The listing builds one solid part. Answer for the finished solid, in the listing's coordinates (mm). Coordinates: 2 decimals unless noted, no trailing zeros. Order: outer loops, then holes, each group sorted by start corner. A loop starts at its lowest first (then second) coordinate and runs counter-clockwise, first axis right, second up. Notation, with made-up numbers: (-18, 13.25) -> (30, 13.25) arc R28 ccw to (30, 35.25) -> close; hole circle Ø11 at (-19.5, 73.25). An arc over 180 degrees is marked (long way). Put each result on its own line as item: value. Start each with the question number.
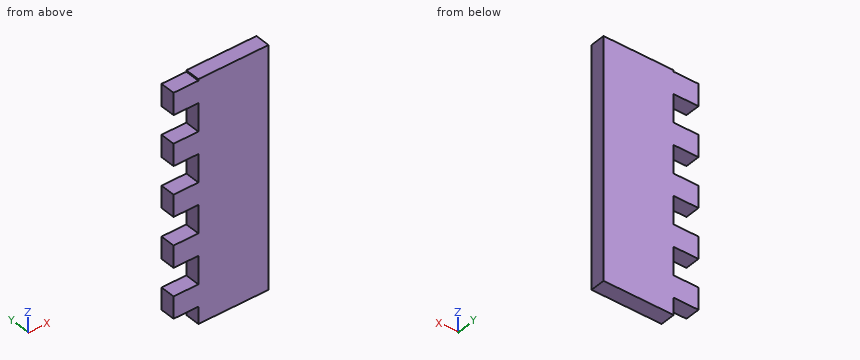
```python
from build123d import *

# Parameters (mm, degrees)
SKETCH_1_W          = 19.1304083
SKETCH_1_H          = 50
EXTRUDE_1_DEPTH     = 3
SKETCH_2_W          = 5
SKETCH_2_H          = 5
CUT_EXTRUDE_1_DEPTH = 3
SKETCH_3_W          = 18.086961025
SKETCH_3_H          = 4.686767273
CUT_EXTRUDE_2_DEPTH = 3
SKETCH_4_W          = 5
SKETCH_4_H          = 0.605391548
CUT_EXTRUDE_3_DEPTH = 10


with BuildPart() as part:
    # 草图1 → 凸台-拉伸1 (new body)
    with BuildSketch(Plane(origin=(0, 0, 0), x_dir=(1, 0, 0), z_dir=(0, 1, 0))):
        Rectangle(SKETCH_1_W, SKETCH_1_H)
    extrude(amount=EXTRUDE_1_DEPTH)

    # 草图2 → 切除-拉伸1 (cut)
    with BuildSketch(Plane(origin=(0, 3, 0), x_dir=(1, 0, 0), z_dir=(0, 1, 0))):
        with Locations((-7.06520415, 12.5)):
            Rectangle(SKETCH_2_W, SKETCH_2_H)
        with Locations((-7.06520415, 22.5)):
            Rectangle(SKETCH_2_W, SKETCH_2_H)
        with Locations((-7.06520415, 2.5)):
            Rectangle(SKETCH_2_W, SKETCH_2_H)
        with Locations((-7.06520415, -7.5)):
            Rectangle(SKETCH_2_W, SKETCH_2_H)
        with Locations((-7.06520415, -17.5)):
            Rectangle(SKETCH_2_W, SKETCH_2_H)
    extrude(amount=-CUT_EXTRUDE_1_DEPTH, mode=Mode.SUBTRACT)

    # 草图3 → 切除-拉伸2 (cut)
    with BuildSketch(Plane(origin=(0, 3, 0), x_dir=(1, 0, 0), z_dir=(0, 1, 0))):
        with Locations((3.01992157, 25.438245622)):
            Rectangle(SKETCH_3_W, SKETCH_3_H)
    extrude(amount=-CUT_EXTRUDE_2_DEPTH, mode=Mode.SUBTRACT)

    # 草图4 → 切除-拉伸3 (cut)
    with BuildSketch(Plane(origin=(0, 3, 0), x_dir=(1, 0, 0), z_dir=(0, 1, 0))):
        with Locations((-7.06520415, 20)):
            Rectangle(SKETCH_4_W, SKETCH_4_H)
        with Locations((-7.06520415, 15)):
            Rectangle(SKETCH_4_W, SKETCH_4_H)
        with Locations((-7.06520415, 5)):
            Rectangle(SKETCH_4_W, SKETCH_4_H)
        with Locations((-7.06520415, 10)):
            Rectangle(SKETCH_4_W, SKETCH_4_H)
        with Locations((-7.06520415, -5)):
            Rectangle(SKETCH_4_W, SKETCH_4_H)
        with Locations((-7.06520415, 0)):
            Rectangle(SKETCH_4_W, SKETCH_4_H)
        with Locations((-7.06520415, -15)):
            Rectangle(SKETCH_4_W, SKETCH_4_H)
        with Locations((-7.06520415, -10)):
            Rectangle(SKETCH_4_W, SKETCH_4_H)
        with Locations((-7.06520415, -25)):
            Rectangle(SKETCH_4_W, SKETCH_4_H)
        with Locations((-7.06520415, -20)):
            Rectangle(SKETCH_4_W, SKETCH_4_H)
    extrude(amount=-CUT_EXTRUDE_3_DEPTH, mode=Mode.SUBTRACT)


solid = part.part
```
(1) The part is cut by section B-B on z = -3.5. Determine the outline of the cut face in (x, y).
(2) The part is cut by section A-A on y = 0.45. Determine the outline of the cut face in (x, z), plus the area to 3 significant figures.
(3) Each of these flat-tipped pins is pushed along its axis until it touches: P1, Ø1.5, axis at x = -6.5, y = 1, coming from the +Z side; P2, Ø0.9, axis at y = 1.5, z = 17, coming from the -X side; P3, Ø0.9, axis at x = -6, y = 1, coming from the -Z side. Where does it stop, or does it pass through?
(4) Find the intervals of material crossed by L1, parallel to Z at x = -8.5, y = 2.5; L2, parallel to X at y = 1.05, z = -10, in increasing order.
Worked out:
1. outline: (-4.57, 0) -> (9.57, 0) -> (9.57, 3) -> (-4.57, 3) -> close
2. outline: (-9.57, -19.7) -> (-4.57, -19.7) -> (-4.57, -23.09) -> (9.57, -23.09) -> (9.57, 25) -> (-4.57, 25) -> (-4.57, 24.7) -> (-9.57, 24.7) -> (-9.57, 20.3) -> (-4.57, 20.3) -> (-4.57, 14.7) -> (-9.57, 14.7) -> (-9.57, 10.3) -> (-4.57, 10.3) -> (-4.57, 4.7) -> (-9.57, 4.7) -> (-9.57, 0.3) -> (-4.57, 0.3) -> (-4.57, -5.3) -> (-9.57, -5.3) -> (-9.57, -9.7) -> (-4.57, -9.7) -> (-4.57, -15.3) -> (-9.57, -15.3) -> close
2. area: 789 mm2
3. P1: z = 24.7
3. P2: x = -4.57
3. P3: z = -19.7
4. L1: -19.7 to -15.3, -9.7 to -5.3, 0.3 to 4.7, 10.3 to 14.7, 20.3 to 24.7
4. L2: -4.57 to 9.57
